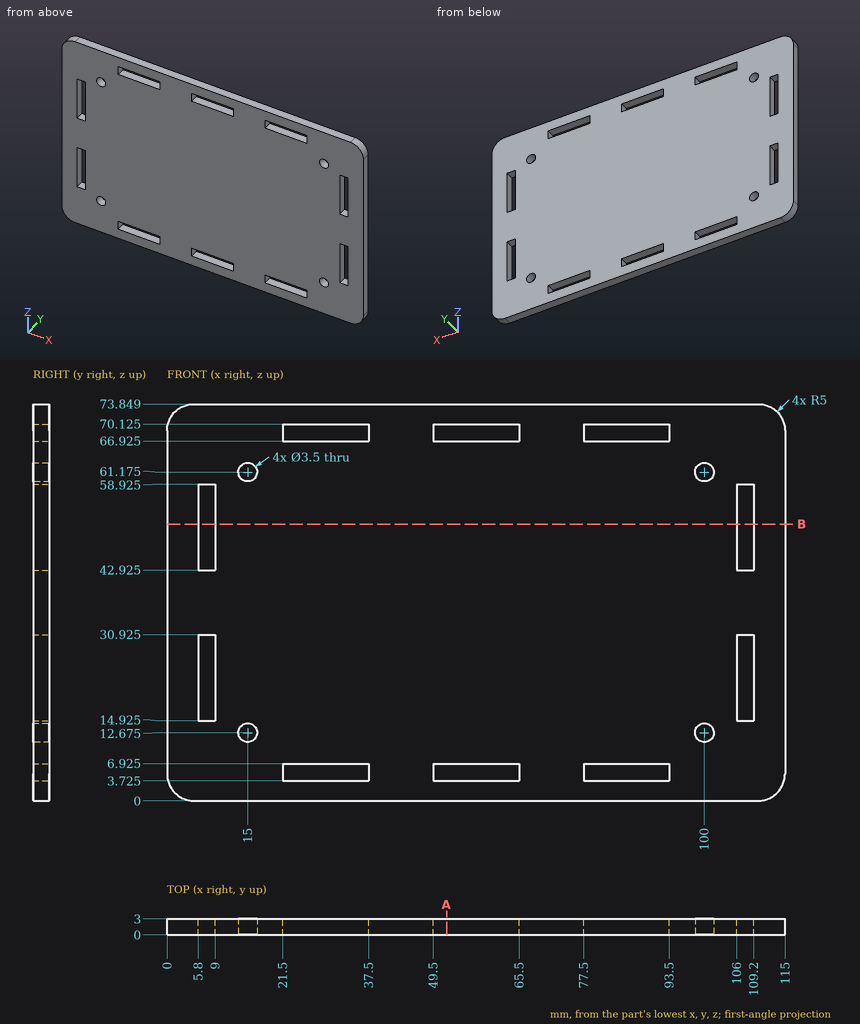
Source: three-view drawing plus pictorial views. Frame: mm from the lowest corner of the part. Give positions to 0.01 mm unless a question says otherwise; leave off trailing zeros. Write each loop counter-clockwise with the first axis right and the second up, starting at its lowest first coordinate (ties: lowest second). Pieces come first, ordered by that corner, then holes.
(1) Cut plane B-B, the plane z = 51.5. Return loops of the section in (x, y).
(2) Cut plane A-A, the plane x = 52. Give the number of separate pieces and of enclosed holes in the cut face, then the cut area to 3 significant figures.
(3) Ray query, line 1 (X direction, y = 0.7, z = 19); line 2 (X direction, y = 1.45, z = 12.5). Return the intervals inside material, ascending.
(4) First-contact query: P1, Ø3, axis at x = 100, z = 12.67, coming from the +Y side. Flat tip, straight axial feed; report the tip coordinate or a pass-through.
Values follow:
1. outline: (0, 0) - (5.8, 0) - (5.8, 3) - (0, 3) - close; (9, 0) - (106, 0) - (106, 3) - (9, 3) - close; (109.2, 0) - (115, 0) - (115, 3) - (109.2, 3) - close
2. separate pieces: 3
2. enclosed holes: 0
2. area: 202 mm2
3. line 1: x = 0 to 5.8, 9 to 106, 109.2 to 115
3. line 2: x = 0 to 13.26, 16.74 to 98.26, 101.74 to 115
4. P1: passes through
